Verification items for the finished model (mm, model axes). Face numbers are marked on the shaded views. A direction names the side the tool comes from. Coordinates: 2 decimals unless noted, no trailing zeros. Order: outer loops, then holes, each group sorted by start corner. A loop starts at its lowest first (then second) coordinate and runs counter-clockwise, first axis right, second up. Notation, with made-up numbers: (70, -31.75) -> (90, -31.75) arc R26 ccw to (90, -4.75) -> close; hole circle Ø6 at (-30.75, 32.5). An arc over 180 degrees is marked (long way). Use CSV: the item, a comma, the result in double quotes. Start each with the question number.
1) Sectioned sample at A-A on x = 5.75. Record the boundary of the cut face in (y, z), then the cut area to 3 significant figures.
2) Tool access check on the marked faces 1, 2 and 3. Record the directions out of +Z, -Z, +X, -X, +Y, -Y that give a thin tool (end or side, any length) a straight path to the whole face; none if there is none.
3) Sectioned sample at B-B on y = 3.25. Record the boundary of the cut face in (x, z), then the cut area to 3 significant figures.
4) Sectioned sample at C-C on z = 9.5. Record the boundary of the cut face in (x, y).
5) Sectioned sample at D-D on x = 11. Record the boundary of the cut face in (y, z), then the cut area to 3 significant figures.
6) Scan lines: line 1 along Z through (x, y) = (10.5, 5); line 2 along Y through (x, z) = (8.5, 1.5); line 3 along X through (y, z) = (4.25, 9). Record each from-to range of solid material in increasing order.
7) Go/stop test with flat-tipped pins: pin 1 (14.5 mm diameter, centred on x = 8, z = 34, fed in from +Y); pin 2 (3.5 mm diameter, centred on y = 3, z = 43.5, fed in from -X); pin 3 (4 mm diameter, centred on y = 5.5, z = 27, fed in from -X). Record where each tip stops, or that it passes through.
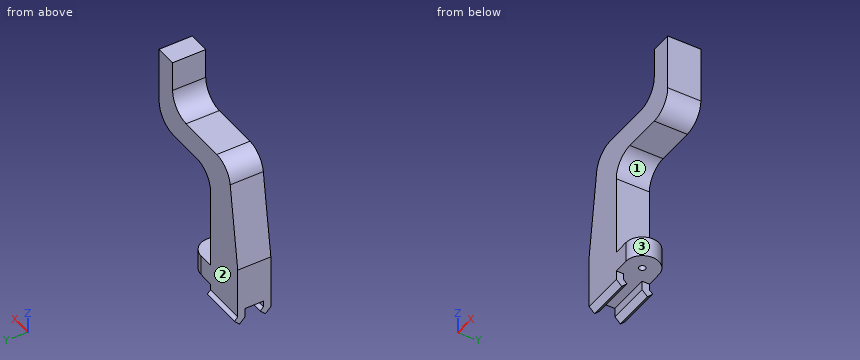
from build123d import *

# Parameters (mm, degrees)
SKETCH2_W           = 10
SKETCH2_H           = 14.768412439
BOSS_EXTRUDE1_DEPTH = 5
BOSS_EXTRUDE4_DEPTH = 10
SKETCH9_W           = 10
SKETCH9_H           = 3.18
SKETCH9_H_2         = 3.888412439
CUT_EXTRUDE3_DEPTH  = 5
BOSS_EXTRUDE5_DEPTH = 7.7
SKETCH12_R          = 0.75
BOSS_EXTRUDE7_DEPTH = 4.75


with BuildPart() as part:
    # Sketch2 → Boss-Extrude1 (new body)
    with BuildSketch(Plane.XY):
        with Locations((0, 1.566049366)):
            Rectangle(SKETCH2_W, SKETCH2_H)
    extrude(amount=BOSS_EXTRUDE1_DEPTH)

    # Sketch8 → Boss-Extrude4 (add)
    with BuildSketch(Plane.ZY.offset(5)):
        Polygon((-0.15, 5.770255585), (0, 5.770255585), (0, 4.070255585), (-0.15, 4.070255585), (-2.137867966, 4.070255585), (-3.402081528, 5.334469147), (-2.2, 6.536550675), (-1.43370491, 5.770255585), align=None)
        Polygon((-0.15, -1.929744415), (0, -1.929744415), (0, -0.229744415), (-0.15, -0.229744415), (-1.43370491, -0.229744415), (-2.2, 0.536550675), (-3.402081528, -0.665530853), (-2.137867966, -1.929744415), align=None)
    extrude(amount=-BOSS_EXTRUDE4_DEPTH)

    # Sketch9 → Cut-Extrude3 (cut)
    with BuildSketch(Plane(origin=(0, 0, 0), x_dir=(-1, 0, 0), z_dir=(0, 0, -1))):
        with Locations((0, 7.360255585)):
            Rectangle(SKETCH9_W, SKETCH9_H)
        with Locations((0, -3.873950635)):
            Rectangle(SKETCH9_W, SKETCH9_H_2)
    extrude(amount=-CUT_EXTRUDE3_DEPTH, mode=Mode.SUBTRACT)

    # Sketch10 → Boss-Extrude5 (add)
    with BuildSketch(Plane(origin=(0, 5.770255585, 0), x_dir=(1, 0, 0), z_dir=(0, 1, 0))):
        with BuildLine():
            Line((-5, -5), (-5, -10.5))
            Line((-5, -10.5), (-2.224545314, -30.248386236))
            ThreePointArc((-2.224545314, -30.248386236), (-0.553500116, -33.326068633), (2.726795029, -34.552520732))
            Line((2.726795029, -34.552520732), (13.995577548, -34.552520732))
            ThreePointArc((13.995577548, -34.552520732), (17.531111453, -36.016986826), (18.995577548, -39.552520732))
            Line((18.995577548, -39.552520732), (18.995577548, -46.600725687))
            Line((18.995577548, -46.600725687), (23.967852608, -46.600725687))
            Line((23.967852608, -46.600725687), (23.967852608, -33.43279758))
            ThreePointArc((23.967852608, -33.43279758), (22.503386514, -29.897263674), (18.967852608, -28.43279758))
            Line((18.967852608, -28.43279758), (10, -28.43279758))
            ThreePointArc((10, -28.43279758), (6.464466094, -26.968331486), (5, -23.43279758))
            Line((5, -23.43279758), (5, -14))
            Line((5, -14), (5, -5))
            Line((5, -5), (-5, -5))
        make_face()
    extrude(amount=-BOSS_EXTRUDE5_DEPTH)

    # Sketch12 → Boss-Extrude7 (add)
    with BuildSketch(Plane.XY):
        with BuildLine():
            Line((5, 5.770255585), (8.5, 5.770255585))
            ThreePointArc((8.5, 5.770255585), (12.35, 1.920255585), (8.5, -1.929744415))
            Line((8.5, -1.929744415), (5, -1.929744415))
            Line((5, -1.929744415), (5, 5.770255585))
        make_face()
        with Locations((8.5, 1.920255585)):
            Circle(SKETCH12_R, mode=Mode.SUBTRACT)
    extrude(amount=BOSS_EXTRUDE7_DEPTH)


solid = part.part
Answers follow:
1,outline,"(-1.93, 0) -> (5.77, 0) -> (5.77, 4.75) -> (-1.93, 4.75) -> close; (-1.93, 26.07) -> (5.77, 26.07) -> (5.77, 34.55) -> (-1.93, 34.55) -> close"
1,area,"102 mm²"
2,face 1,"+X, +Y, -Y"
2,face 2,"+Z, +X, -X, +Y"
2,face 3,"-Z, +X"
3,outline,"(-5, 0) -> (12.11, 0) -> (12.11, 4.75) -> (5, 4.75) -> (5, 23.43) arc R5 cw to (10, 28.43) -> (18.97, 28.43) arc R5 ccw to (23.97, 33.43) -> (23.97, 46.6) -> (19, 46.6) -> (19, 39.55) arc R5 cw to (14, 34.55) -> (2.73, 34.55) arc R5 ccw to (-2.22, 30.25) -> (-5, 10.5) -> close"
3,area,"516 mm²"
4,outline,"(-5, -1.93) -> (5, -1.93) -> (5, 5.77) -> (-5, 5.77) -> close"
5,outline,"(-1.93, 28.43) -> (5.77, 28.43) -> (5.77, 34.55) -> (-1.93, 34.55) -> close; (-1.01, 0) -> (4.85, 0) -> (4.85, 4.75) -> (-1.01, 4.75) -> close"
5,area,"74.9 mm²"
6,line 1,"z = 0 to 4.75, 28.43 to 34.55"
6,line 2,"y = -1.93 to 1.17, 2.67 to 5.77"
6,line 3,"x = -5 to 5"
7,pin 1,"stops at y = 5.77"
7,pin 2,"stops at x = 19"
7,pin 3,"stops at x = -2.96"
